Check sheet for the modelled part. Datum: model origin and axes. Units: mm. Coordinates: 2 decimals unless noted, no trailing zeros. Write each loop counter-clockwise with the first axis right and the second up, starting at its lowest first coordinate (ties: lowest second). Pieces come first, ordered by that corner, then holes. Notation, with made-up numbers: (22.25, 14) -> (33.25, 14) arc R30 ccw to (33.25, 36) -> close; hole circle Ø11 at (40.5, 61.5). An arc over 180 degrees is marked (long way). Put each result on its own line as item: value.
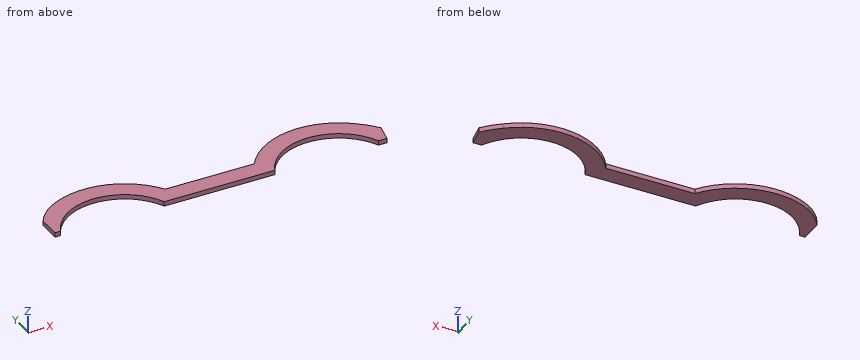
```python
from build123d import *

# Parameters (mm, degrees)
BOSS_EXTRUDE1_DEPTH = 3


with BuildPart() as part:
    # Sketch1 → Boss-Extrude1 (new body)
    with BuildSketch(Plane.XY):
        with BuildLine():
            Line((-5.630682288, 0), (0, 0))
            Line((0, 0), (2.527819158, 12))
            ThreePointArc((2.527819158, 12), (-2.1947123, 17.496295373), (-7.549171204, 22.379054435))
            ThreePointArc((-7.549171204, 22.379054435), (-46.881030658, 34.019398375), (-81.487950058, 12))
            Line((-81.487950058, 12), (-140.512049942, 12))
            ThreePointArc((-140.512049942, 12), (-171.177028416, 33.302311395), (-208, 27.121847063))
            ThreePointArc((-208, 27.121847063), (-214.715828047, 21.616866872), (-220, 14.725954012))
            Line((-220, 14.725954012), (-220, 0))
            Line((-220, 0), (-216.369317712, 0))
            ThreePointArc((-216.369317712, 0), (-182, 22.5), (-147.630682288, 0))
            Line((-147.630682288, 0), (-74.369317712, 0))
            ThreePointArc((-74.369317712, 0), (-40, 22.5), (-5.630682288, 0))
        make_face()
    extrude(amount=BOSS_EXTRUDE1_DEPTH)


solid = part.part
```
Q1. Cross-section at C-C (x = -110.5). Record the cut outline in (y, z).
Recorded:
outline: (0, 0) -> (12, 0) -> (12, 3) -> (0, 3) -> close
Q2. Material ranges on line 1 along X through (y, z) = (10, 1.55); line 2 along X through (y, z) = (12.5, 2.25); line 3 along X through (y, z) = (6.5, 1.4), recorded low to high.
Recorded:
line 1: x = -220 to -209.95, -154.05 to -67.95, -12.05 to 2.11
line 2: x = -220 to -207.5, -156.5 to -140.84, -81.16 to -65.5, -14.5 to 2.14
line 3: x = -220 to -212.72, -151.28 to -70.72, -9.28 to 1.37
Q3. Cross-section at B-B (y = 31.5). Record the cut outline in (x, z).
Recorded:
outline: (-198.97, 0) -> (-165.03, 0) -> (-165.03, 3) -> (-198.97, 3) -> close; (-56.97, 0) -> (-23.03, 0) -> (-23.03, 3) -> (-56.97, 3) -> close
Q4. Cross-section at A-A (z = 2.35). Record the cut outline in (x, y).
Recorded:
outline: (-220, 0) -> (-216.37, 0) arc R37.5 cw to (-147.63, 0) -> (-74.37, 0) arc R37.5 cw to (-5.63, 0) -> (0, 0) -> (2.53, 12) arc R59.62 ccw to (-7.55, 22.38) arc R49.5 ccw to (-81.49, 12) -> (-140.51, 12) arc R49.5 ccw to (-208, 27.12) arc R37.84 ccw to (-220, 14.73) -> close
Q5. Cross-section at D-D (x = -192). Record the cut outline in (y, z), plus the area to 3 significant figures.
Recorded:
outline: (21.14, 0) -> (33.48, 0) -> (33.48, 3) -> (21.14, 3) -> close
area: 37.0 mm2
Q6. Depth check by flat-ended pin: P1, Ø1.5, axis at x = -125, z = 1, coming from the +Y side; P2, Ø5, axis at x = -124.5, y = 16, coming from the +Z side. Enter the tip coordinate at first touch or a pass-through.
Recorded:
P1: stops at y = 12
P2: passes through
